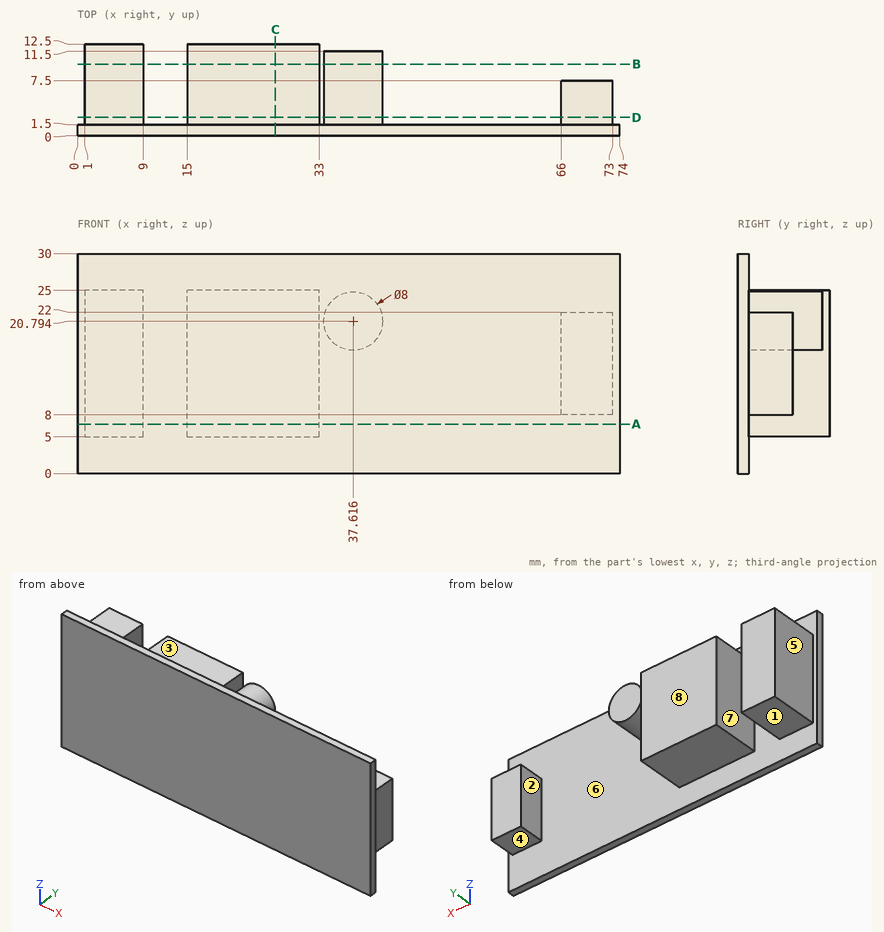
For this review, use the dimensioned drawing (mm, ordinates from the lowest corner) and the shaded views. A direction names the side the tool comes from. Coordinates: 2 decimals unless noted, no trailing zeros. Write each loop counter-clockwise with the first axis right and the second up, starting at its lowest first coordinate (ties: lowest second). Pieces come first, ordered by that corner, then holes. Notation, with made-up numbers: (-27.75, 88.5) -> (14.25, 88.5) arc R27 cw to (14.25, 107.5) -> close; hole circle Ø4 at (82.25, 20.25). An arc over 180 degrees is marked (long way). Put each result on its own line as item: value.
Q1. The part is to be moulded in two halves that separate along X. For the marked faces 5, 6, 7 and 8, say which applies: +X half, -X half, draft (parallel to the pull), parting line (faces both ways), or undercut.
From the geometry:
face 5: -X half
face 6: undercut
face 7: undercut
face 8: draft
Q2. Take a section at C-C, the plane x = 27. State the section outline as (y, z) points.
From the geometry:
outline: (0, 0) -> (1.5, 0) -> (1.5, 5) -> (12.5, 5) -> (12.5, 25) -> (1.5, 25) -> (1.5, 30) -> (0, 30) -> close
Q3. Tool access review of the marked faces 1, 2, 3 and 4: name each direction out of +Z, -Z, +X, -X, +Y, -Y from which nothing blocks a thin tool from reaching the whole face with its end or side.
From the geometry:
face 1: -Z, +X, -X, +Y
face 2: +Z, -Z, +Y
face 3: +Z, +X, -X, +Y
face 4: -Z, +X, +Y
Q4. Take a section at A-A, the plane z = 6.75. State the section outline as (x, y) points.
From the geometry:
outline: (0, 0) -> (74, 0) -> (74, 1.5) -> (33, 1.5) -> (33, 12.5) -> (15, 12.5) -> (15, 1.5) -> (9, 1.5) -> (9, 12.5) -> (1, 12.5) -> (1, 1.5) -> (0, 1.5) -> close
Q5. Wall thickness on L1, parallel to X at y = 8.5, z = 10.5; L2, parallel to X at y = 8.75, z = 23 (1 decimal); L3, parallel to X at y = 5.25, z = 23.25 (1 decimal): over which ranges is each line inside the solid? List them lowest first.
From the geometry:
L1: x = 1 to 9, 15 to 33
L2: x = 1 to 9, 15 to 33, 34.3 to 41
L3: x = 1 to 9, 15 to 33, 34.5 to 40.8
Q6. Clearance check with flat-ended pins moving along their axes: pin 1 Ø1.8 at (x, y) = (69.5, 4.5) entering from -Z; pin 2 Ø8 at (x, z) = (52, 12.5) entering from +Y; pin 3 Ø6.5 at (x, y) = (3, 9) entering from +Z. State where each tip first meets the part, or that it passes through.
From the geometry:
pin 1: stops at z = 8
pin 2: stops at y = 1.5
pin 3: stops at z = 25
Q7. Take a section at D-D, the plane y = 2.5. State the section outline as (x, z) points (1 decimal), then the cut area to 3 significant figures.
From the geometry:
outline: (1, 5) -> (9, 5) -> (9, 25) -> (1, 25) -> close; (15, 5) -> (33, 5) -> (33, 25) -> (15, 25) -> close; circle Ø8 at (37.6, 20.8); (66, 8) -> (73, 8) -> (73, 22) -> (66, 22) -> close
area: 668 mm2
Q8. Take a section at B-B, the plane y = 9.75. State the section outline as (x, z) points (1 decimal), then the cut area to 3 significant figures.
From the geometry:
outline: (1, 5) -> (9, 5) -> (9, 25) -> (1, 25) -> close; (15, 5) -> (33, 5) -> (33, 25) -> (15, 25) -> close; circle Ø8 at (37.6, 20.8)
area: 570 mm2
